```python
from build123d import *

# Parameters (mm, degrees)
BASE_FLANGE1_DEPTH      = 78
EDGE_FLANGE1_DEPTH      = 22
EDGE_FLANGE1_BEND_DEPTH = 22
SKETCH14_R              = 2.25
CUT_EXTRUDE1_DEPTH      = 33
SKETCH15_R              = 6.75
CUT_EXTRUDE2_DEPTH      = 85.599054368
CUT_EXTRUDE3_DEPTH      = 88.475710915
CUT_EXTRUDE3_DEPTH_BACK = 88.475710915
SKETCH16_R              = 2


# Sheet-metal steps are written as plain solids
with BuildPart() as part:
    # Sketch3 → Base-Flange1 (new body)
    with BuildSketch(Plane(origin=(0, 0, 0), x_dir=(0, 0, -1), z_dir=(1, 0, 0))):
        with BuildLine():
            Line((-20, 14), (-3, 14))
            ThreePointArc((-3, 14), (-0.878679656, 13.121320344), (0, 11))
            Line((0, 11), (0, -11))
            ThreePointArc((0, -11), (-0.878679656, -13.121320344), (-3, -14))
            Line((-3, -14), (-20, -14))
            Line((-20, -14), (-20, -13))
            Line((-20, -13), (-3, -13))
            ThreePointArc((-3, -13), (-1.585786438, -12.414213562), (-1, -11))
            Line((-1, -11), (-1, 11))
            ThreePointArc((-1, 11), (-1.585786438, 12.414213562), (-3, 13))
            Line((-3, 13), (-20, 13))
            Line((-20, 13), (-20, 14))
        make_face()
    extrude(amount=BASE_FLANGE1_DEPTH)

    # Edge-Flange1 section (across the edge) → Edge-Flange1 (add)
    with BuildSketch(Plane(origin=(80, 11, 0), x_dir=(-1, 0, 0), z_dir=(0, -1, 0))):
        with BuildLine():
            Line((-1, 2), (-1, 20))
            Line((-1, 20), (0, 20))
            Line((0, 20), (0, 2))
            ThreePointArc((0, 2), (0.585786438, 0.585786438), (2, 0))
            Line((2, 0), (2, -1))
            ThreePointArc((2, -1), (-0.121320344, -0.121320344), (-1, 2))
        make_face()
    extrude(amount=EDGE_FLANGE1_DEPTH)

    # Edge-Flange1 section 2 (across the edge) → Edge-Flange1 bend (add)
    with BuildSketch(Plane(origin=(-2, -11, 0), x_dir=(1, 0, 0), z_dir=(0, 1, 0))):
        with BuildLine():
            Line((-1, 2), (-1, 20))
            Line((-1, 20), (0, 20))
            Line((0, 20), (0, 2))
            ThreePointArc((0, 2), (0.585786438, 0.585786438), (2, 0))
            Line((2, 0), (2, -1))
            ThreePointArc((2, -1), (-0.121320344, -0.121320344), (-1, 2))
        make_face()
    extrude(amount=EDGE_FLANGE1_BEND_DEPTH)

    # Sketch14 → Cut-Extrude1 (cut)
    with BuildSketch(Plane(origin=(0, 14, 0), x_dir=(1, 0, 0), z_dir=(0, 1, 0))):
        with Locations(Location((16, -11, 0), (0, 0, 270))):
            Circle(SKETCH14_R)
        with Locations(Location((62, -11, 0), (0, 0, 270))):
            Circle(SKETCH14_R)
    extrude(amount=-CUT_EXTRUDE1_DEPTH, mode=Mode.SUBTRACT)

    # Sketch15 → Cut-Extrude2 (cut, through all)
    with BuildSketch(Plane(origin=(0, 0, 0), x_dir=(-1, 0, 0), z_dir=(0, 0, -1))):
        with Locations((-39, 0)):
            Circle(SKETCH15_R)
    extrude(amount=-CUT_EXTRUDE2_DEPTH, mode=Mode.SUBTRACT)

    # Sketch16 → Cut-Extrude3 (cut, two sides: drawn at the far end of the back side and taken through both)
    with BuildSketch(Plane.ZY.offset(3).offset(-CUT_EXTRUDE3_DEPTH_BACK)):
        with Locations((-15, 5)):
            Circle(SKETCH16_R)
        with Locations((-7.5, 5)):
            Circle(SKETCH16_R)
        with Locations((-7.5, -6.338473389)):
            Circle(SKETCH16_R)
        with Locations((-15, -6.338473389)):
            Circle(SKETCH16_R)
    extrude(amount=CUT_EXTRUDE3_DEPTH + CUT_EXTRUDE3_DEPTH_BACK, mode=Mode.SUBTRACT)


solid = part.part
```
Can you work these out from the model? Positions are in its coordinate system, mm. A direction names the side the tool comes from. Coordinates: 2 decimals unless noted, no trailing zeros. Loops run counter-clockwise (first coordinate to the right, second up) from the corner with the lowest first, then second, coordinate; pieces in that order, holes last.
1) Imagine slicing it at B-B on x = 39. List the corners of the cut face in (y, z) for me, plus the area to 3 significant figures.
2) For pin 1 (3.5 mm diameter, centred on x = -1.5, z = -12.5, fed in from -Y); pin 2 (10 mm diameter, centred on x = 70, y = -7.5, fed in from -Z); pin 3 (2 mm diameter, centred on x = 15.5, y = 7.5, fed in from +Z), each with a flat end and sliding along its axis, tell me the tip position at first contact or that it passes through.
3) Imagine slicing it at D-D on z = -15. List the corners of the cut face in (x, y) for me.
4) Which directions (+Z, -Z, +X, -X, +Y, -Y) give clear straight access to the entire face, cutting with the end or side of a thin tool? Please do faces 5 (the flat face through (78, -13.15, 7.64)), 6 (the flat face through (-2, 0, -11)), 7 (the flat face through (38, 13, 11)).
5) I need wall thicknesses on probe 1 along Y at (x, z) = (80.3, -15); probe 2 along X at (y, z) = (-7.25, -3.5); probe 3 along Y at (x, z) = (38.5, 7.5). Which ranges of each line are inside material? Lowest first, please.
6) Thinking about a two-plate mould opening in Y: for faces 1 (the flat face through (-2.4, 11, -9.5)), 2 (the flat face through (78, 13.2, 7.6)), 3 (the cylindrical face through (-2.493, 5.088, -9.498)), 4 (the cylindrical face through (-2.5, -6.3, -9.5)), which applies, pulls with the +Y half, pulls with the -Y half, needs draft (parallel to the pull), parting line crosses it, or undercut?
7) Imagine slicing it at C-C on x = 62. List the corners of the cut face in (y, z) for me.
8) Imagine slicing it at A-A on z = 5. List the corners of the cut face in (x, y) for me.
Completed:
1. outline: (-14, 3) arc R3 ccw to (-11, 0) - (-6.75, 0) - (-6.75, 1) - (-11, 1) arc R2 cw to (-13, 3) - (-13, 20) - (-14, 20) - close; (6.75, 0) - (11, 0) arc R3 ccw to (14, 3) - (14, 20) - (13, 20) - (13, 3) arc R2 cw to (11, 1) - (6.75, 1) - close
1. area: 50.4 mm2
2. pin 1: stops at y = -11
2. pin 2: stops at z = 0
2. pin 3: stops at z = 1
3. outline: (-3, -11) - (-2, -11) - (-2, -8.34) - (-3, -8.34) - close; (-3, -4.34) - (-2, -4.34) - (-2, 3) - (-3, 3) - close; (-3, 7) - (-2, 7) - (-2, 11) - (-3, 11) - close; (80, -11) - (81, -11) - (81, -8.34) - (80, -8.34) - close; (80, -4.34) - (81, -4.34) - (81, 3) - (80, 3) - close; (80, 7) - (81, 7) - (81, 11) - (80, 11) - close
4. face 5: +Z, -Z, +X, -Y
4. face 6: -Z, +Y, -Y
4. face 7: +Z, +X, -X
5. probe 1: y = -11 to -8.34, -4.34 to 3, 7 to 11
5. probe 2: x = -3 to -2, 80 to 81
5. probe 3: y = -14 to -13, 13 to 14
6. face 1: pulls with the +Y half
6. face 2: needs draft
6. face 3: undercut
6. face 4: undercut
7. outline: (-14, 3) arc R3 ccw to (-11, 0) - (11, 0) arc R3 ccw to (14, 3) - (14, 8.75) - (13, 8.75) - (13, 3) arc R2 cw to (11, 1) - (-11, 1) arc R2 cw to (-13, 3) - (-13, 8.75) - (-14, 8.75) - close; (-14, 13.25) - (-13, 13.25) - (-13, 20) - (-14, 20) - close; (13, 13.25) - (14, 13.25) - (14, 20) - (13, 20) - close
8. outline: (0, -14) - (78, -14) - (78, -13) - (0, -13) - close; (0, 13) - (78, 13) - (78, 14) - (0, 14) - close
